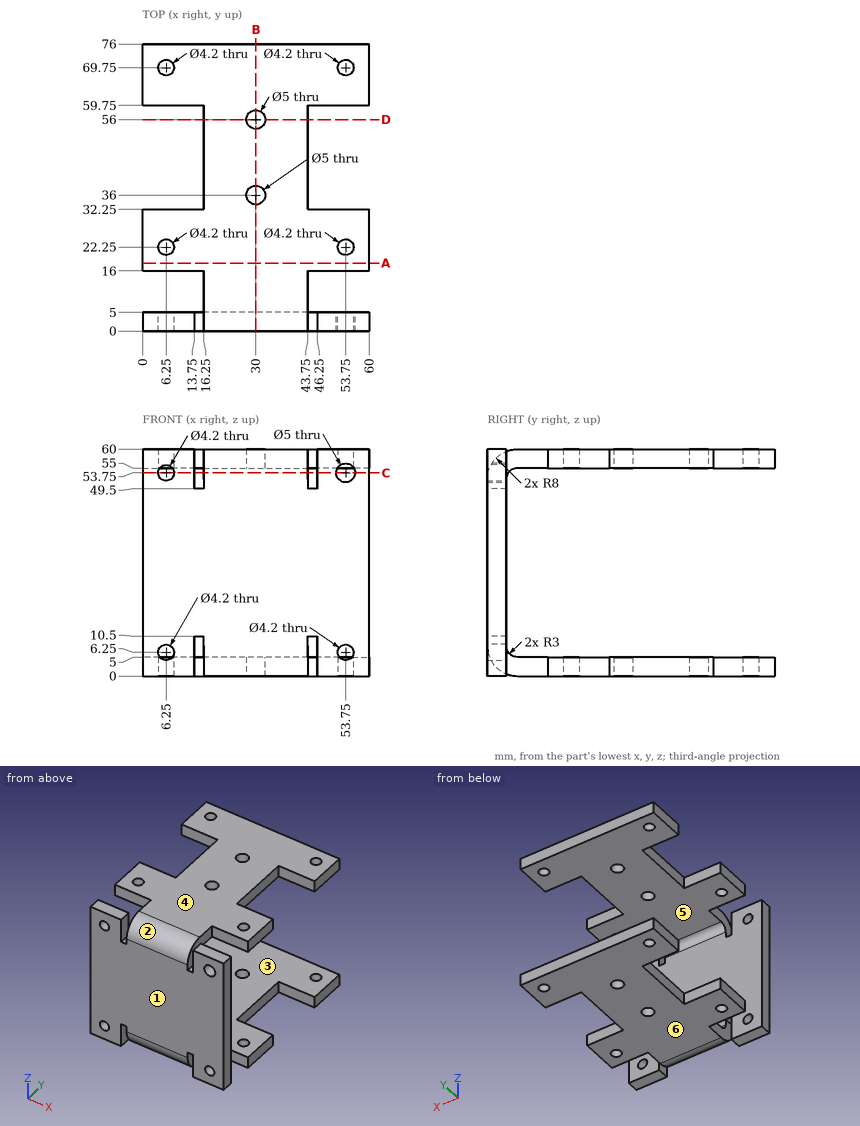
Job drawing, mm, ordinate dimensions from the low corner. One solid piece. A direction names the side the tool comes from. Round coordinates to 2 decimals unless told otherwise and drop trailing zeros. Write each loop counter-clockwise with the first axis right and the second up, starting at its lowest first coordinate (ties: lowest second). Pieces come first, ordered by that corner, then holes. Notation, with made-up numbers: M 54.5,55.25 L 104.5,55.25 A22 cw 104.5,89.25 Z; hole C -4,8.5 d10. An arc over 180 degrees is marked long. Return JSON: item names as keys, results as strings. Group by question number.
(1) Which spindle directions (+Z, -Z, +X, -X, +Y, -Y) get a long thin tool onto all of the face, cutting with end or side? Do the marked faces 1, 2 and 3. Say none if no direction does.
(2) Pin check, flat tips, straight feed: pin 1 Ø10 at (x, z) = (46, 34.5) entering from +Y; pin 2 Ø5.5 at (y, z) = (40, 58) entering from -X; pin 3 Ø1.2 at (x, y) = (45.5, 2.5) entering from +Z. Stop position of each tip, or through.
(3) Drill centre lines: probe 1 along Y at (x, z) = (53.75, 1.4); probe 2 along X at (y, z) = (3.65, 6.25); probe 3 along X at (y, z) = (22.25, 1.45). Where is each one in solid material? Low to high.
(4) Two-plate mould, pull along Z, no slides. Class the marked faces 4, 5 and 6: +Z half, -Z half, draft (parallel to the pull), parting line (faces both ways), or undercut.
(5) Saw through at D-D on y = 56. Write the cut outline in (x, z).
(6) Saw through at B-B on x = 30. Write the cut outline in (y, z), then the cut area to 3 significant figures.
(7) Saw through at C-C on z = 53.75. Write the cut outline in (x, y).
(8) Saw through at A-A on y = 18. Write the cut outline in (x, z), then the cut area to 3 significant figures.
Returned:
{
 "1": {"face 1": "+Z, -Z, +X, -X, -Y", "face 2": "+Z, -Y", "face 3": "+X, -X, +Y"},
 "2": {"pin 1": "y = 5", "pin 2": "x = 16.25", "pin 3": "z = 49.5"},
 "3": {"probe 1": "0 to 5, 16 to 20.15, 24.35 to 32.25, 59.75 to 67.65, 71.85 to 76", "probe 2": "0 to 4.15, 8.35 to 13.75, 16.25 to 43.75, 46.25 to 51.65, 55.85 to 60", "probe 3": "0 to 4.15, 8.35 to 51.65, 55.85 to 60"},
 "4": {"face 4": "+Z half", "face 5": "undercut", "face 6": "-Z half"},
 "5": {"outline": "M 16.25,0 L 27.5,0 L 27.5,5 L 16.25,5 Z; M 16.25,55 L 27.5,55 L 27.5,60 L 16.25,60 Z; M 32.5,0 L 43.75,0 L 43.75,5 L 32.5,5 Z; M 32.5,55 L 43.75,55 L 43.75,60 L 32.5,60 Z"},
 "6": {"outline": "M 0,8 A8 ccw 8,0 L 33.5,0 L 33.5,5 L 8,5 A3 cw 5,8 L 5,52 A3 cw 8,55 L 33.5,55 L 33.5,60 L 8,60 A8 ccw 0,52 Z; M 38.5,0 L 53.5,0 L 53.5,5 L 38.5,5 Z; M 38.5,55 L 53.5,55 L 53.5,60 L 38.5,60 Z; M 58.5,0 L 76,0 L 76,5 L 58.5,5 Z; M 58.5,55 L 76,55 L 76,60 L 58.5,60 Z", "area": "886 mm²"},
 "7": {"outline": "M 0,0 L 4.15,0 L 4.15,5 L 0,5 Z; M 8.35,0 L 13.75,0 L 13.75,5 L 8.35,5 Z; M 16.25,0.19 L 43.75,0.19 L 43.75,5.56 L 16.25,5.56 Z; M 46.25,0 L 51.25,0 L 51.25,5 L 46.25,5 Z; M 56.25,0 L 60,0 L 60,5 L 56.25,5 Z"},
 "8": {"outline": "M 0,0 L 60,0 L 60,5 L 0,5 Z; M 0,55 L 60,55 L 60,60 L 0,60 Z", "area": "600 mm²"}
}
